Check sheet for the modelled part. Datum: model origin and axes. Units: mm. Round coordinates to 2 decimals unless told otherwise and drop trailing zeros. Write each loop counter-clockwise with the first axis right and the second up, starting at its lowest first coordinate (ties: lowest second). Pieces come first, ordered by that corner, then holes. Notation, with made-up numbers: (60, -29) -> (114, -29) arc R6 ccw to (114, -24) -> close; hole circle Ø7 at (22.25, 42.5). An arc over 180 degrees is marked (long way). One line per item, written item: value. Start each with the question number.
```python
from build123d import *

# Parameters (mm, degrees)
SKETCH_1_W          = 30
SKETCH_1_H          = 60
EXTRUDE_1_DEPTH     = 10
SKETCH_2_R          = 2
CUT_EXTRUDE_1_DEPTH = 40


with BuildPart() as part:
    # 草图1 → 凸台-拉伸1 (new body)
    with BuildSketch(Plane(origin=(0, 0, 0), x_dir=(1, 0, 0), z_dir=(0, 1, 0))):
        Rectangle(SKETCH_1_W, SKETCH_1_H)
    extrude(amount=EXTRUDE_1_DEPTH)

    # 草图2 → 切除-拉伸1 (cut)
    with BuildSketch(Plane(origin=(0, 0, -30), x_dir=(-1, 0, 0), z_dir=(0, 0, -1))):
        with Locations((-7.5, 5)):
            Circle(SKETCH_2_R)
        with Locations(Location((7.5, 5, 0), (0, 0, 180))):
            Circle(SKETCH_2_R)
    extrude(amount=-CUT_EXTRUDE_1_DEPTH, mode=Mode.SUBTRACT)


solid = part.part
```
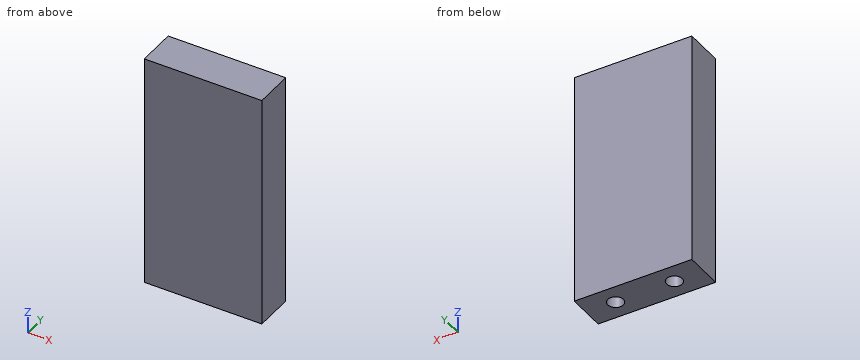
1. Cross-section at B-B (z = 7). Record the cut outline in (x, y), plus the area to 3 significant figures.
2. Cross-section at A-A (x = -7.5). Record the cut outline in (y, z), plus the area to 3 significant figures.
3. Depth check by flat-ended pin: pin 1 Ø1.5 at (x, z) = (2.5, 9) entering from -Y. Enter the tip coordinate at first touch or a pass-through.
4. Material ranges on probe 1 along Y at (x, z) = (-7.5, -5.5); probe 2 along Z at (x, y) = (8.5, 5), recorded low to high.
5. Cross-section at C-C (y = 5). Record the cut outline in (x, z).
Working result:
1. outline: (-15, 0) -> (15, 0) -> (15, 10) -> (-15, 10) -> close; hole circle Ø4 at (-7.5, 5); hole circle Ø4 at (7.5, 5)
1. area: 275 mm^2
2. outline: (0, -30) -> (3, -30) -> (3, 10) -> (7, 10) -> (7, -30) -> (10, -30) -> (10, 30) -> (0, 30) -> close
2. area: 440 mm^2
3. pin 1: stops at y = 0
4. probe 1: y = 0 to 3, 7 to 10
4. probe 2: z = 10 to 30
5. outline: (-15, -30) -> (-9.5, -30) -> (-9.5, 10) -> (-5.5, 10) -> (-5.5, -30) -> (5.5, -30) -> (5.5, 10) -> (9.5, 10) -> (9.5, -30) -> (15, -30) -> (15, 30) -> (-15, 30) -> close
